```python
from build123d import *

# Parameters (mm, degrees)
SKETCH1_R           = 1.7
BOSS_EXTRUDE1_DEPTH = 5
SKETCH2_R           = 2.3
BOSS_EXTRUDE2_DEPTH = 2.85
SKETCH3_W           = 9
SKETCH3_H           = 0.7
BOSS_EXTRUDE3_DEPTH = 3.1


with BuildPart() as part:
    # Sketch1 → Boss-Extrude1 (new body, symmetric)
    with BuildSketch(Plane.XY):
        with BuildLine():
            Line((2, 0), (26, 0))
            ThreePointArc((26, 0), (27.414213562, 0.585786438), (28, 2))
            Line((28, 2), (28, 14))
            ThreePointArc((28, 14), (27.414213562, 15.414213562), (26, 16))
            Line((26, 16), (2, 16))
            ThreePointArc((2, 16), (0.585786438, 15.414213562), (0, 14))
            Line((0, 14), (0, 2))
            ThreePointArc((0, 2), (0.585786438, 0.585786438), (2, 0))
        make_face()
        with Locations((3.8, 2.9)):
            Circle(SKETCH1_R, mode=Mode.SUBTRACT)
        with Locations((24.2, 13.1)):
            Circle(SKETCH1_R, mode=Mode.SUBTRACT)
    extrude(amount=BOSS_EXTRUDE1_DEPTH, both=True)

    # Sketch2 → Boss-Extrude2 (add, symmetric)
    with BuildSketch(Plane.XY):
        with BuildLine():
            Line((16.443613757, 17.263612158), (15.919001734, 12.923377494))
            Line((15.919001734, 12.923377494), (16.415388776, 12.863378293))
            Line((16.415388776, 12.863378293), (17, 17.7))
            Line((17, 17.7), (7.504443651, 18.847745091))
            Line((7.504443651, 18.847745091), (7.690168637, 20.384290169))
            ThreePointArc((7.690168637, 20.384290169), (6.024003677, 19.933239209), (4.513291566, 20.768285054))
            Line((4.513291566, 20.768285054), (4.267567379, 18.735352933))
            Line((4.267567379, 18.735352933), (16.443613757, 17.263612158))
        make_face()
        with Locations((6.3, 22.216619605)):
            Circle(SKETCH2_R)
    extrude(amount=BOSS_EXTRUDE2_DEPTH, both=True)

    # Sketch3 → Boss-Extrude3 (add, symmetric)
    with BuildSketch(Plane.XY):
        with Locations((32.5, 10.35)):
            Rectangle(SKETCH3_W, SKETCH3_H)
        with Locations((32.5, 5.65)):
            Rectangle(SKETCH3_W, SKETCH3_H)
        Polygon((15.6, 0), (15.6, -3.4), (24.2, -3.4), (24.2, -2.7), (16.3, -2.7), (16.3, 0), align=None)
    extrude(amount=BOSS_EXTRUDE3_DEPTH, both=True)


solid = part.part
```
CAD build for the part. Positions are in the model's coordinates, mm. A direction names the side the tool comes from. Give positions to 0.01 mm unless a question says otherwise; leave off trailing zeros. Loops run counter-clockwise (first coordinate to the right, second up) from the corner with the lowest first, then second, coordinate; pieces in that order, holes last. Notation, with made-up numbers: (1, 16.25) - (37, 16.25) arc R11 ccw to (37, 25.25) - close; hole circle Ø5 at (-18, -20). An arc over 180 degrees is marked (long way). Put each result on its own line as item: value.
Q1. Slice it at A-A (z = 3.5). Give the cut face in (x, y), plus the area to 3 significant figures.
Filled in:
outline: (0, 2) arc R2 ccw to (2, 0) - (26, 0) arc R2 ccw to (28, 2) - (28, 14) arc R2 ccw to (26, 16) - (2, 16) arc R2 ccw to (0, 14) - close; hole circle Ø3.4 at (3.8, 2.9); hole circle Ø3.4 at (24.2, 13.1)
area: 426 mm²
Q2. Tool access for faces 5 (the face through (32, 5.3, 0)), 6 (the face through (10.27, 18.01, 0.04)), 7 (the face through (20, -3.4, 0)): list every direction of +Z, -Z, +X, -X, +Y, -Y with a clear straight run to the whole face (end or side of a thin tool).
Filled in:
face 5: +Z, -Z, +X, -Y
face 6: +Z, -Z, -X
face 7: +Z, -Z, +X, -X, -Y
Q3. Probe line 1 along Y through (x, z) = (3.8, -2); line 2 along Y through (x, z) = (21.5, -2.5); line 3 along Y through (x, z) = (16, 3). List the from-to ranges inside material, lowest first.
Filled in:
line 1: y = 0 to 1.2, 4.6 to 16
line 2: y = -3.4 to -2.7, 0 to 16
line 3: y = -3.4 to 16
Q4. Slice it at D-D (z = 1.25). Give the number of separate pieces and of enclosed holes in the cut face, plus the area to 3 significant figures.
Filled in:
separate pieces: 1
enclosed holes: 2
area: 474 mm²
Q5. Slice it at B-B (x = 20.5). Give the cut face in (y, z), plus the area to 3 significant figures.
Filled in:
outline: (-3.4, -3.1) - (-2.7, -3.1) - (-2.7, 3.1) - (-3.4, 3.1) - close; (0, -5) - (16, -5) - (16, 5) - (0, 5) - close
area: 164 mm²
Q6. Flat gauge pins, fed straight in: pin 1 (2.5 mm diameter, centred on x = 12, y = 20.5, fed in from -Z); pin 2 (3 mm diameter, centred on x = 32, z = 0, fed in from +Y); pin 3 (0.8 mm diameter, centred on x = 32.5, y = 10, fed in from -Z); pin 4 (1.5 mm diameter, centred on x = 13.5, y = 17.5, fed in from -Z). Where does each tip first touch, or does it go through?
Filled in:
pin 1: passes through
pin 2: stops at y = 10.7
pin 3: stops at z = -3.1
pin 4: stops at z = -2.85
Q7. Mould opens along Y. For faces 1 (the face through (32, 6, 0)), 2 (the face through (32, 10.7, 0)), 3 (the face through (16.3, -1, 0)), 4 (the face through (8, 21, -2.85)) say: pulls with the +Y half, pulls with the -Y half, needs draft (parallel to the pull), parting line crosses it, or undercut.
Filled in:
face 1: undercut
face 2: pulls with the +Y half
face 3: undercut
face 4: needs draft
Q8. Slice it at C-C (y = 13.1). Give the cut face in (x, z), plus the area to 3 significant figures.
Filled in:
outline: (0, -5) - (22.5, -5) - (22.5, 5) - (0, 5) - close; (25.9, -5) - (28, -5) - (28, 5) - (25.9, 5) - close
area: 246 mm²
